For this review, take the finished solid that the model builds, in its own axes (mm). A direction names the side the tool comes from. Coordinates: 2 decimals unless noted, no trailing zeros. Order: outer loops, then holes, each group sorted by start corner. A loop starts at its lowest first (then second) coordinate and runs counter-clockwise, first axis right, second up. Notation, with made-up numbers: (70.25, 25) -> (84.25, 25) arc R22 cw to (84.25, 40) -> close; hole circle Ø2 at (77.5, -18.75). An arc over 180 degrees is marked (long way). Answer as a JSON object with one key per item and string values. Group by question number.
1) For pin 1 (2 mm diameter, centred on x = -30, z = -21.65, fed in from +Y), flat-tipped, find the tip position at first contact; note if it passes through.
2) Draft analysis for pull direction Z (two halves, no side actions). For faces 1 (the flat face through (-32.5, -7, -9)), 2 (the flat face through (-17, 0, -6)), 3 (the conical face through (27.364, -14.957, -6.516)), state which applies: +Z half, -Z half, draft (parallel to the pull), parting line (faces both ways), or undercut.
3) Wall thickness on L1, parallel to Z at x = -27, y = -22.5; L2, parallel to Y at x = 0, z = -9.25; L3, parallel to X at y = -25, z = -21: over which ranges is each line inside the solid? List them lowest first.
4) Add section C-C, the plane z = -27.5. Write out the cut boundary in (x, y) (3 decimals).
5) Add section A-A, the plane z = -17. Write out the cut boundary in (x, y), then the cut area to 3 significant figures.
6) Machinability: for faces 4 (the cylindrical face through (-25, 0, -3)), 5 (the flat face through (17, 21, -13)), 6 (the flat face through (30.04, -15.28, -22.86)), 7 (the cylindrical face through (24.595, 25.93, -6.021)), 8 (the cylindrical face through (-29.1, -23.4, -6.59)), which of the approach directions +Z, -Z, +X, -X, +Y, -Y give a long, thin tool a straight path to every point of the face, cutting with its end or side? Answer none if there is none.
7) Add section B-B, the plane x = 0. Write out the cut boundary in (y, z).
from build123d import *

# Parameters (mm, degrees)
SKETCH1_W                       = 65
SKETCH1_H                       = 62
BOSS_EXTRUDE1_DEPTH             = 13
BOSS_EXTRUDE2_REACH             = 48.757
BOSS_EXTRUDE2_DIRECTION_2_REACH = 48.757
SKETCH3_W                       = 55
SKETCH3_H                       = 20
CUT_EXTRUDE1_DEPTH              = 56.733742024
SKETCH5_R                       = 16
CUT_EXTRUDE3_DEPTH              = 56.733742024
SKETCH4_R                       = 26
CUT_EXTRUDE2_DEPTH              = 7
SKETCH6_R                       = 2.5
CUT_EXTRUDE4_DEPTH              = 56.733742024
FILLET1_R                       = 0.5
TAP_DRILL_FOR_M5X0_8_TAP1_D     = 4.2
TAP_DRILL_FOR_M5X0_8_TAP1_DEPTH = 15
TAP_DRILL_FOR_M5X0_8_TAP1_TIP   = 1.2618073
TAP_DRILL_FOR_M3X0_5_TAP1_D     = 2.5
TAP_DRILL_FOR_M3X0_5_TAP1_DEPTH = 10
TAP_DRILL_FOR_M3X0_5_TAP1_TIP   = 0.751075774
TAP_DRILL_FOR_M3X0_5_TAP2_D     = 2.5
TAP_DRILL_FOR_M3X0_5_TAP2_DEPTH = 10
TAP_DRILL_FOR_M3X0_5_TAP2_TIP   = 0.751075774


with BuildPart() as part:
    # Sketch1 → Boss-Extrude1 (new body)
    with BuildSketch(Plane.XY):
        Rectangle(SKETCH1_W, SKETCH1_H)
    extrude(amount=-BOSS_EXTRUDE1_DEPTH)

    # Boss-Extrude2: up to this face of the body (flat: up to its plane)
    boss_extrude2_end = Plane(part.part.faces().sort_by_distance((32.5, 0, -6.5))[0])
    # Sketch2 → Boss-Extrude2 (add, up to the picked face)
    with BuildSketch(Plane(origin=(0, 0, 0), x_dir=(0, 0, -1), z_dir=(1, 0, 0)), mode=Mode.PRIVATE) as boss_extrude2_sk1:
        Polygon((13, 0), (33, -31), (13, -31), align=None)
    boss_extrude2_tool1 = split(extrude(boss_extrude2_sk1.sketch, amount=BOSS_EXTRUDE2_REACH, mode=Mode.PRIVATE), bisect_by=boss_extrude2_end, keep=Keep.BOTH, mode=Mode.PRIVATE)
    add(boss_extrude2_tool1.solids().sort_by(Axis((0, -20.666667, -19.666667), (1, 0, 0)))[0])

    # Boss-Extrude2 direction 2: up to this face of the body (flat: up to its plane)
    boss_extrude2_direction_2_end = Plane(part.part.faces().sort_by_distance((-32.5, 0, -6.5))[0])
    # Sketch2 → Boss-Extrude2 direction 2 (add, up to the picked face)
    with BuildSketch(Plane(origin=(0, 0, 0), x_dir=(0, 0, -1), z_dir=(1, 0, 0)), mode=Mode.PRIVATE) as boss_extrude2_direction_2_sk1:
        Polygon((13, 0), (33, -31), (13, -31), align=None)
    boss_extrude2_direction_2_tool1 = split(extrude(boss_extrude2_direction_2_sk1.sketch, amount=-BOSS_EXTRUDE2_DIRECTION_2_REACH, mode=Mode.PRIVATE), bisect_by=boss_extrude2_direction_2_end, keep=Keep.BOTH, mode=Mode.PRIVATE)
    add(boss_extrude2_direction_2_tool1.solids().sort_by(Axis((0, -20.666667, -19.666667), (-1, 0, 0)))[0])

    # Sketch3 → Cut-Extrude1 (cut, through all)
    with BuildSketch(Plane(origin=(0, 0, 0), x_dir=(1, 0, 0), z_dir=(0, 1, 0))):
        with Locations((0, 23)):
            Rectangle(SKETCH3_W, SKETCH3_H)
    extrude(amount=-CUT_EXTRUDE1_DEPTH, mode=Mode.SUBTRACT)

    # Sketch5 → Cut-Extrude3 (cut, through all)
    with BuildSketch(Plane.XY):
        Circle(SKETCH5_R)
    extrude(amount=-CUT_EXTRUDE3_DEPTH, mode=Mode.SUBTRACT)

    # Sketch4 → Cut-Extrude2 (cut)
    with BuildSketch(Plane(origin=(0, 0, -13), x_dir=(-1, 0, 0), z_dir=(0, 0, -1))):
        Circle(SKETCH4_R)
    extrude(amount=-CUT_EXTRUDE2_DEPTH, mode=Mode.SUBTRACT)

    # Sketch6 → Cut-Extrude4 (cut, through all)
    with BuildSketch(Plane.XY):
        with Locations((0, 22.5)):
            Circle(SKETCH6_R)
        with Locations((22.5, 0)):
            Circle(SKETCH6_R)
        with Locations((0, -22.5)):
            Circle(SKETCH6_R)
        with Locations((-22.5, 0)):
            Circle(SKETCH6_R)
    extrude(amount=-CUT_EXTRUDE4_DEPTH, mode=Mode.SUBTRACT)

    # Fillet1
    fillet1_edges = [part.edges().sort_by_distance(p)[0] for p in [
        (26, 0, -13),
        (26, 0, -6),
        (-16, 0, -6),
    ]]
    fillet(fillet1_edges, radius=FILLET1_R)

    # Tap Drill for M5x0.8 Tap1
    with Locations(Plane(origin=(0, -31, 0), x_dir=(-1, 0, 0), z_dir=(0, -1, 0))):
        with Locations((27, 6.5), (-27, 6.5)):
            Hole(TAP_DRILL_FOR_M5X0_8_TAP1_D / 2, depth=TAP_DRILL_FOR_M5X0_8_TAP1_DEPTH)
            with Locations((0, 0, -(TAP_DRILL_FOR_M5X0_8_TAP1_DEPTH + TAP_DRILL_FOR_M5X0_8_TAP1_TIP / 2))):  # 118° drill point
                Cone(0, TAP_DRILL_FOR_M5X0_8_TAP1_D / 2, TAP_DRILL_FOR_M5X0_8_TAP1_TIP, mode=Mode.SUBTRACT)

    # Tap Drill for M3x0.5 Tap1
    with Locations(Plane(origin=(0, -31, 0), x_dir=(-1, 0, 0), z_dir=(0, -1, 0))):
        with Locations((30, 21.65), (-30, 21.65)):
            Hole(TAP_DRILL_FOR_M3X0_5_TAP1_D / 2, depth=TAP_DRILL_FOR_M3X0_5_TAP1_DEPTH)
            with Locations((0, 0, -(TAP_DRILL_FOR_M3X0_5_TAP1_DEPTH + TAP_DRILL_FOR_M3X0_5_TAP1_TIP / 2))):  # 118° drill point
                Cone(0, TAP_DRILL_FOR_M3X0_5_TAP1_D / 2, TAP_DRILL_FOR_M3X0_5_TAP1_TIP, mode=Mode.SUBTRACT)

    # Tap Drill for M3x0.5 Tap2
    with Locations(Plane(origin=(0, 31, 0), x_dir=(1, 0, 0), z_dir=(0, 1, 0))):
        with Locations((25.75, 6.5), (-25.75, 6.5)):
            Hole(TAP_DRILL_FOR_M3X0_5_TAP2_D / 2, depth=TAP_DRILL_FOR_M3X0_5_TAP2_DEPTH)
            with Locations((0, 0, -(TAP_DRILL_FOR_M3X0_5_TAP2_DEPTH + TAP_DRILL_FOR_M3X0_5_TAP2_TIP / 2))):  # 118° drill point
                Cone(0, TAP_DRILL_FOR_M3X0_5_TAP2_D / 2, TAP_DRILL_FOR_M3X0_5_TAP2_TIP, mode=Mode.SUBTRACT)


solid = part.part
Output values:
{
 "1": {"pin 1": "stops at y = -11.86"},
 "2": {"face 1": "draft", "face 2": "-Z half", "face 3": "undercut"},
 "3": {"L1": "z = -13 to -8.6, -4.4 to 0", "L2": "y = -31 to -26, 26 to 31", "L3": "x = -32.5 to -31.07, -28.93 to -27.5, 27.5 to 28.93, 31.07 to 32.5"},
 "4": {"outline": "(-32.5, -31) -> (-27.5, -31) -> (-27.5, -22.475) -> (-32.5, -22.475) -> close; (27.5, -31) -> (32.5, -31) -> (32.5, -22.475) -> (27.5, -22.475) -> close"},
 "5": {"outline": "(-32.5, -31) -> (-27.5, -31) -> (-27.5, -6.2) -> (-32.5, -6.2) -> close; (27.5, -31) -> (32.5, -31) -> (32.5, -6.2) -> (27.5, -6.2) -> close", "area": "248 mm²"},
 "6": {"face 4": "+Z, -Z", "face 5": "-Z, +Y", "face 6": "-Z, +X, -X, +Y", "face 7": "+Y", "face 8": "-Y"},
 "7": {"outline": "(-31, -13) -> (-26.5, -13) arc R0.5 ccw to (-26, -12.5) -> (-26, -6.5) arc R0.5 cw to (-25.5, -6) -> (-25, -6) -> (-25, 0) -> (-31, 0) -> close; (-20, -6) -> (-16.5, -6) arc R0.5 ccw to (-16, -5.5) -> (-16, 0) -> (-20, 0) -> close; (16, -5.5) arc R0.5 ccw to (16.5, -6) -> (20, -6) -> (20, 0) -> (16, 0) -> close; (25, -6) -> (25.5, -6) arc R0.5 cw to (26, -6.5) -> (26, -12.5) arc R0.5 ccw to (26.5, -13) -> (31, -13) -> (31, 0) -> (25, 0) -> close"}
}
